Verification items for this drawing (mm, ordinates from the low corner). Give positions to 0.01 mm unless a question says otherwise; leave off trailing zeros. Loops run counter-clockwise (first coordinate to the right, second up) from the corner with the lowest first, then second, coordinate; pieces in that order, holes last. Notation, with made-up numbers: (35.25, -20) -> (85.25, -20) arc R27 ccw to (85.25, 5) -> close; hole circle Ø4 at (56.25, 22). An arc over 180 degrees is marked (long way). Use one line per item in the form item = value. Start each with the question number.
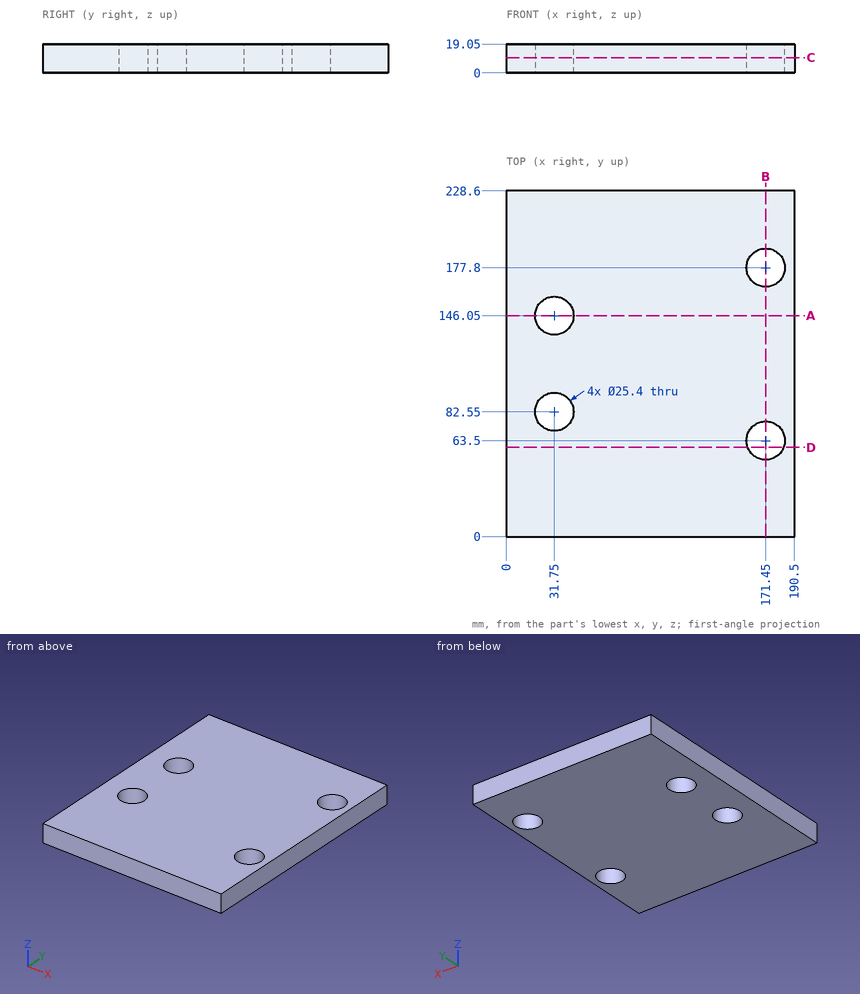
Item 1: Sectioned sample at D-D, the plane y = 59. Enter the section's corners in (x, z).
Item 2: Sectioned sample at B-B, the plane x = 171.45. Enter the section's corners in (y, z), and give its area (3 significant figures).
Item 3: Gauge pin test, flat end, axial feed: pin 1 Ø20.5 at (x, y) = (31.75, 146.05) entering from -Z. Record the tip position at first contact, or that the pin passes through.
Item 4: Material ranges on line 1 (Y direction, x = 31.75, z = 6.25); line 2 (Y direction, x = 172, z = 4); line 3 (X direction, y = 171, z = 10.5), recorded low to high.
Item 5: Sectioned sample at A-A, the plane y = 146.05. Enter the section's corners in (x, z), and give its area (3 significant figures).
Item 6: Sectioned sample at C-C, the plane z = 10. Enter the section's corners in (x, y).
Outcome:
q1.outline = (0, 0) -> (159.57, 0) -> (159.57, 19.05) -> (0, 19.05) -> close; (183.33, 0) -> (190.5, 0) -> (190.5, 19.05) -> (183.33, 19.05) -> close
q2.outline = (0, 0) -> (50.8, 0) -> (50.8, 19.05) -> (0, 19.05) -> close; (76.2, 0) -> (165.1, 0) -> (165.1, 19.05) -> (76.2, 19.05) -> close; (190.5, 0) -> (228.6, 0) -> (228.6, 19.05) -> (190.5, 19.05) -> close
q2.area = 3,390 mm^2
q3.pin_1 = through
q4.line_1 = 0 to 69.85, 95.25 to 133.35, 158.75 to 228.6
q4.line_2 = 0 to 50.81, 76.19 to 165.11, 190.49 to 228.6
q4.line_3 = 0 to 160.72, 182.18 to 190.5
q5.outline = (0, 0) -> (19.05, 0) -> (19.05, 19.05) -> (0, 19.05) -> close; (44.45, 0) -> (190.5, 0) -> (190.5, 19.05) -> (44.45, 19.05) -> close
q5.area = 3,150 mm^2
q6.outline = (0, 0) -> (190.5, 0) -> (190.5, 228.6) -> (0, 228.6) -> close; hole circle Ø25.4 at (31.75, 82.55); hole circle Ø25.4 at (31.75, 146.05); hole circle Ø25.4 at (171.45, 63.5); hole circle Ø25.4 at (171.45, 177.8)
